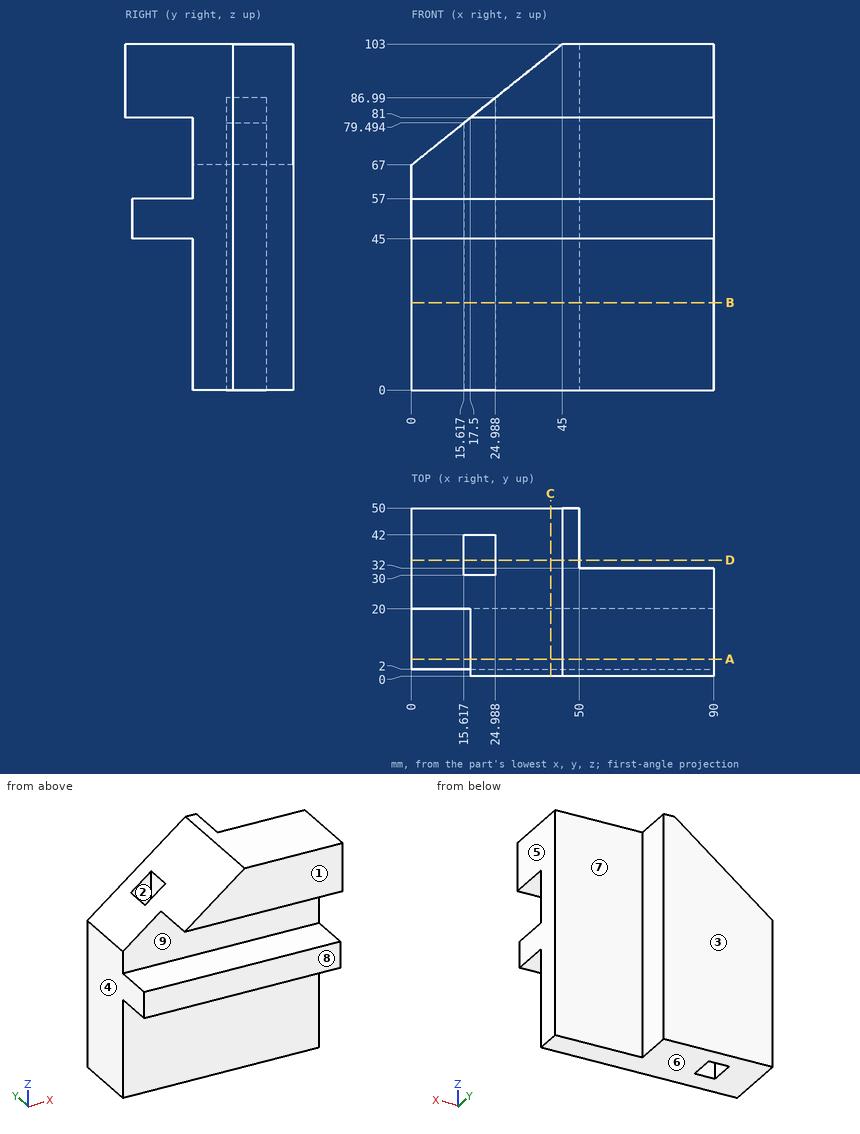
Study the drawing (mm; zero at the part's minimum x, y, z) and answer. A direction names the side the tool comes from. Coordinates: 2 decimals unless noted, no trailing zeros. Loops run counter-clockwise (first coordinate to the right, second up) from the corner with the lowest first, then second, coordinate; pieces in that order, holes last. Notation, with made-up numbers: (41, 21.5) -> (58, 21.5) arc R25 cw to (58, 41.5) -> close; hole circle Ø5 at (14.25, 40.25). An arc over 180 degrees is marked (long way). Answer as CSV lines item,"result".
1) Flat-ended cylindrical pins translate along their axes: pin 1 (10 mm diameter, centred on x = 69.5, z = 31.5, fed in from +Y); pin 2 (5.5 mm diameter, centred on y = 39, z = 46, fed in from +X); pin 3 (4 mm diameter, centred on x = 29, y = 7, fed in from -Z); pin 4 (1.5 mm diameter, centred on x = 64, y = 33, fed in from -Z). Find the tip coordinate at first contact, or state that the pin passes through.
A:
pin 1,"stops at y = 32"
pin 2,"stops at x = 50"
pin 3,"stops at z = 45"
pin 4,"passes through"
2) Straight lines are drawn through the part: probe 1 along Z at (x, y) = (71, 6); probe 2 along X at (y, z) = (35, 25.5); probe 3 along X at (y, z) = (46, 18.5). For each, find the intervals that lie inside material, in ascending order.
A:
probe 1,"z = 45 to 57, 81 to 103"
probe 2,"x = 0 to 15.62, 24.99 to 50"
probe 3,"x = 0 to 50"
3) For the marked faces 5, 6, 7, 8 and 9, determine the directions among +Z, -Z, +X, -X, +Y, -Y from which every point of the face is accessible in a straight line to the end or side of a thin tool.
A:
face 5,"+Z, -Z, +X, +Y, -Y"
face 6,"-Z, +X, -X, +Y, -Y"
face 7,"+Z, -Z, +X, +Y"
face 8,"-Z, +X, -X, -Y"
face 9,"+X, -X, -Y"
4) The part is cut by section A-A (y = 5). Give the vertices of the cut face in (x, z), and give its area (3 significant figures).
A:
outline,"(0, 45) -> (90, 45) -> (90, 57) -> (0, 57) -> close; (17.5, 81) -> (90, 81) -> (90, 103) -> (45, 103) -> close"
area,"2,370 mm²"
5) For a pull along Y with two mould halves and no side action, classify the marked faces 1, 2, 3 and 4 as released by +Y, released by -Y, zero draft, split by the parting line, or undercut.
A:
face 1,"released by -Y"
face 2,"undercut"
face 3,"released by +Y"
face 4,"zero draft"
6) The part is cut by section D-D (y = 34.5). Give the vertices of the cut face in (x, z).
A:
outline,"(0, 0) -> (15.62, 0) -> (15.62, 79.49) -> (0, 67) -> close; (24.99, 0) -> (50, 0) -> (50, 103) -> (45, 103) -> (24.99, 86.99) -> close"
7) The part is cut by section C-C (x = 41.5). Give the vertices of the cut face in (y, z), and give its area (3 significant figures).
A:
outline,"(0, 81) -> (20, 81) -> (20, 57) -> (2, 57) -> (2, 45) -> (20, 45) -> (20, 0) -> (50, 0) -> (50, 100.2) -> (0, 100.2) -> close"
area,"3,610 mm²"
8) The part is cut by section B-B (z = 26). Give the vertices of the cut face in (x, y).
A:
outline,"(0, 20) -> (90, 20) -> (90, 32) -> (50, 32) -> (50, 50) -> (0, 50) -> close; hole (15.62, 30) -> (24.99, 30) -> (24.99, 42) -> (15.62, 42) -> close"
